Can you work these out from the model? Positions are in its coordinate system, mm. A direction names the side the tool comes from. Coordinates: 2 decimals unless noted, no trailing zeros. Order: outer loops, then holes, each group sorted by start corner. A loop starts at its lowest first (then second) coordinate and runs counter-clockwise, first axis right, second up. Notation, with made-up numbers: (24.5, -3.5) - (53.5, -3.5) arc R35 cw to (53.5, 31.5) - close; hole circle Ø9 at (9.25, 55.25). An arc over 180 degrees is marked (long way). Use a Markdown table: item, result. Add a question column.
(1) We'd pull the mould along Y, two halves only. Please class faces 1 (the flat face through (-35, -1, 2)), 2 (the cylindrical face through (-23.199, -38.857, 15.846)), 3 (the cylindrical face through (21.95, -31.42, 13.31)), 4 (the cylindrical face through (0.77, -74.99, 2.46)): pulls with the +Y half, pulls with the -Y half, needs draft (parallel to the pull), parting line crosses it, or undercut.
(2) I want a section at D-D (z = 2). List the corners of the cut face in (x, y) for me.
(3) I want a section at B-B (z = 10). List the corners of the cut face in (x, y) for me, and give its area (3 significant figures).
(4) On a 3-axis mill with a long thin cutter (end or side, diameter ignored), from which of +Z, -Z, +X, -X, +Y, -Y can I reach the whole of each face in a straight line? I mean faces 5 (the cylindrical face through (-27.05, 34.58, 13.31)), 6 (the cylindrical face through (25.801, -38.857, 15.846)). Say none if no direction works.
(5) I want a section at A-A (y = 33). List the corners of the cut face in (x, z) for me.
(6) I want a section at C-C (x = -24.5). List the corners of the cut face in (y, z) for me (3 decimals), and give its area (3 significant figures).
(7) For pin 1 Ø10 at (x, y) = (13, -32) entering from -Z; pin 2 Ø1 at (x, z) = (-23, 12.5) entering from -Y; pin 3 Ø10 at (x, y) = (14, -12) entering from +Z; pin 4 Ø1 at (x, z) = (23, 18.5) entering from +Y, each with a flat end and sliding along its axis, tell me the tip position at first contact or that it passes through.
(8) If I drill on L1, parallel to X at y = 33, z = 19.5; L2, parallel to Y at x = -24.5, z = 12.75; L3, parallel to Z at x = -6, y = 17, over which ranges is the centre line in solid material (lowest first)? Write a range as [from, to].
Autodesk Fusion 360 part; units mm, degrees
sketch "Sketch1" plane through (0, 0, 0) normal (0, 0, 1) x (1, 0, 0)
  line L0 (35, 40) -> (35, -40)
  line L1 (-35, -40) -> (-35, 40)
  line L2 (0, 1.75) -> (0, 22.5)
  line L3 (1.75, 0) -> (22.5, 0)
  arc A0 (-35, -40) -> (35, -40) centre (0, -40) ccw
  arc A1 (35, 40) -> (-35, 40) centre (0, 40) ccw
  dimension "d2" = 80
  dimension "d3" = 70
extrude "Extrude1" add sketch "Sketch1" along normal blind 5
sketch "Sketch2" plane through (0, 0, 5) normal (0, 0, 1) x (-1, 0, 0)
  arc A0 (35, 40) -> (-35, 40) centre (0, 40) ccw
  line L0 (-35, 40) -> (-35, -40)
  arc A1 (-35, -40) -> (35, -40) centre (0, -40) ccw
  line L1 (35, -40) -> (35, 40)
  line L2 (24.5, -33) -> (-24.5, -33) construction
  line L3 (-24.5, -33) -> (-24.5, 33) construction
  line L4 (-24.5, 33) -> (24.5, 33) construction
  line L5 (24.5, 33) -> (24.5, -33) construction
  line L6 (-1.75, 0) -> (-22.5, 0)
  line L7 (0, -1.75) -> (0, -22.5)
  point P0 (24.5, -33)
  point P1 (-24.5, -33)
  point P2 (-24.5, 33)
  point P3 (24.5, 33)
  dimension "d6" = 49
  dimension "d7" = 66
hole "Hole1" at (-24.5, 33, 5) at (24.5, 33, 5) at (24.5, -33, 5) at (-24.5, -33, 5) direction (0, 0, -1) diameter 6 end through all
sketch "Sketch3" plane through (0, 0, 5) normal (0, 0, 1) x (-1, 0, 0)
  circle A0 centre (-24.5, 33) radius 3
  circle A1 centre (24.5, -33) radius 3
  circle A2 centre (-24.5, -33) radius 3
  circle A3 centre (24.5, 33) radius 3
  arc A4 (35, 40) -> (-35, 40) centre (0, 40) ccw
  line L0 (-35, 40) -> (-35, -40)
  arc A5 (-35, -40) -> (35, -40) centre (0, -40) ccw
  line L1 (35, -40) -> (35, 40)
  circle A6 centre (24.5, -33) radius 3
  circle A7 centre (-24.5, -33) radius 3
  circle A8 centre (-24.5, 33) radius 3
  circle A9 centre (24.5, 33) radius 3
  circle A10 centre (24.5, -33) radius 6
  circle A11 centre (-24.5, -33) radius 6
  circle A12 centre (24.5, 33) radius 6
  circle A13 centre (-24.5, 33) radius 6
  dimension "d10" = 3
  dimension "d11" = 3
  dimension "d12" = 3
  dimension "d13" = 3
extrude "Extrude2" add sketch "Sketch3" along normal blind 22 contours A10 | A11 | A12 | A13
Answers follow:
| question | item | result |
|---|---|---|
| 1 | face 1 | needs draft |
| 1 | face 2 | undercut |
| 1 | face 3 | undercut |
| 1 | face 4 | pulls with the -Y half |
| 2 | outline | (-35, -40) arc R35 ccw to (35, -40) - (35, 40) arc R35 ccw to (-35, 40) - close; hole circle Ø6 at (-24.5, -33); hole circle Ø6 at (-24.5, 33); hole circle Ø6 at (24.5, -33); hole circle Ø6 at (24.5, 33) |
| 3 | outline | circle Ø12 at (-24.5, -33); circle Ø12 at (-24.5, 33); circle Ø12 at (24.5, -33); circle Ø12 at (24.5, 33); hole circle Ø6 at (-24.5, -33); hole circle Ø6 at (-24.5, 33); hole circle Ø6 at (24.5, -33); hole circle Ø6 at (24.5, 33) |
| 3 | area | 339 mm² |
| 4 | face 5 | +Z, -Z |
| 4 | face 6 | +Z |
| 5 | outline | (-35, 0) - (-27.5, 0) - (-27.5, 27) - (-30.5, 27) - (-30.5, 5) - (-35, 5) - close; (-21.5, 0) - (21.5, 0) - (21.5, 27) - (18.5, 27) - (18.5, 5) - (-18.5, 5) - (-18.5, 27) - (-21.5, 27) - close; (27.5, 0) - (35, 0) - (35, 5) - (30.5, 5) - (30.5, 27) - (27.5, 27) - close |
| 6 | outline | (-64.995, 0) - (-36, 0) - (-36, 27) - (-39, 27) - (-39, 5) - (-64.995, 5) - close; (-30, 0) - (30, 0) - (30, 27) - (27, 27) - (27, 5) - (-27, 5) - (-27, 27) - (-30, 27) - close; (36, 0) - (64.995, 0) - (64.995, 5) - (39, 5) - (39, 27) - (36, 27) - close |
| 6 | area | 854 mm² |
| 7 | pin 1 | stops at z = 0 |
| 7 | pin 2 | stops at y = -38.92 |
| 7 | pin 3 | stops at z = 5 |
| 7 | pin 4 | stops at y = 38.92 |
| 8 | L1 | x = [-30.5, -27.5], [-21.5, -18.5], [18.5, 21.5], [27.5, 30.5] |
| 8 | L2 | y = [-39, -36], [-30, -27], [27, 30], [36, 39] |
| 8 | L3 | z = [0, 5] |
